from build123d import *

# Parameters (mm, degrees)
SKETCH2_R           = 4.1
SKETCH2_R_2         = 2.6
BOSS_EXTRUDE1_DEPTH = 5


with BuildPart() as part:
    # Sketch2 → Boss-Extrude1 (new body)
    # profile 1 of 2: a face of its own
    with BuildSketch(Plane.XY):
        with BuildLine():
            ThreePointArc((-8.388352144, 2.232508627), (-7.643352144, 2.753972912), (-8.388352144, 3.275437196))
            Line((-8.388352144, 3.275437196), (-8.388352144, 4.232508627))
            ThreePointArc((-8.388352144, 4.232508627), (-7.805907881, 4.361528648), (-7.67688786, 4.943972912))
            Line((-7.67688786, 4.943972912), (-6.719816429, 4.943972912))
            ThreePointArc((-6.719816429, 4.943972912), (-6.198352144, 4.198972912), (-5.67688786, 4.943972912))
            Line((-5.67688786, 4.943972912), (-4.719816429, 4.943972912))
            ThreePointArc((-4.719816429, 4.943972912), (-4.198352144, 4.198972912), (-3.67688786, 4.943972912))
            Line((-3.67688786, 4.943972912), (-2.719816429, 4.943972912))
            ThreePointArc((-2.719816429, 4.943972912), (-2.198352144, 4.198972912), (-1.67688786, 4.943972912))
            Line((-1.67688786, 4.943972912), (-0.719816429, 4.943972912))
            ThreePointArc((-0.719816429, 4.943972912), (-0.198352144, 4.198972912), (0.32311214, 4.943972912))
            Line((0.32311214, 4.943972912), (1.280183571, 4.943972912))
            ThreePointArc((1.280183571, 4.943972912), (1.409203592, 4.361528648), (1.991647856, 4.232508627))
            Line((1.991647856, 4.232508627), (1.991647856, 3.275437196))
            ThreePointArc((1.991647856, 3.275437196), (1.246647856, 2.753972912), (1.991647856, 2.232508627))
            Line((1.991647856, 2.232508627), (1.991647856, 1.275437196))
            ThreePointArc((1.991647856, 1.275437196), (1.246647856, 0.753972912), (1.991647856, 0.232508627))
            Line((1.991647856, 0.232508627), (1.991647856, -0.724562804))
            ThreePointArc((1.991647856, -0.724562804), (1.246647856, -1.246027088), (1.991647856, -1.767491373))
            Line((1.991647856, -1.767491373), (1.991647856, -2.724562804))
            ThreePointArc((1.991647856, -2.724562804), (1.246647856, -3.246027088), (1.991647856, -3.767491373))
            Line((1.991647856, -3.767491373), (1.991647856, -4.724562804))
            ThreePointArc((1.991647856, -4.724562804), (1.409203592, -4.853582824), (1.280183571, -5.436027088))
            Line((1.280183571, -5.436027088), (0.32311214, -5.436027088))
            ThreePointArc((0.32311214, -5.436027088), (-0.198352144, -4.691027088), (-0.719816429, -5.436027088))
            Line((-0.719816429, -5.436027088), (-1.67688786, -5.436027088))
            ThreePointArc((-1.67688786, -5.436027088), (-2.198352144, -4.691027088), (-2.719816429, -5.436027088))
            Line((-2.719816429, -5.436027088), (-3.67688786, -5.436027088))
            ThreePointArc((-3.67688786, -5.436027088), (-4.198352144, -4.691027088), (-4.719816429, -5.436027088))
            Line((-4.719816429, -5.436027088), (-5.67688786, -5.436027088))
            ThreePointArc((-5.67688786, -5.436027088), (-6.198352144, -4.691027088), (-6.719816429, -5.436027088))
            Line((-6.719816429, -5.436027088), (-7.67688786, -5.436027088))
            ThreePointArc((-7.67688786, -5.436027088), (-7.805907881, -4.853582824), (-8.388352144, -4.724562804))
            Line((-8.388352144, -4.724562804), (-8.388352144, -3.767491373))
            ThreePointArc((-8.388352144, -3.767491373), (-7.643352144, -3.246027088), (-8.388352144, -2.724562804))
            Line((-8.388352144, -2.724562804), (-8.388352144, -1.767491373))
            ThreePointArc((-8.388352144, -1.767491373), (-7.643352144, -1.246027088), (-8.388352144, -0.724562804))
            Line((-8.388352144, -0.724562804), (-8.388352144, 0.232508627))
            ThreePointArc((-8.388352144, 0.232508627), (-7.643352144, 0.753972912), (-8.388352144, 1.275437196))
            Line((-8.388352144, 1.275437196), (-8.388352144, 2.232508627))
        make_face()
        with Locations((-3.198352144, -0.246027088)):
            Circle(SKETCH2_R, mode=Mode.SUBTRACT)
    # profile 2 of 2: a face of its own
    with BuildSketch(Plane.XY):
        with Locations((-3.198352144, -0.246027088)):
            Circle(SKETCH2_R)
        with Locations((-3.198352144, -0.246027088)):
            Circle(SKETCH2_R_2, mode=Mode.SUBTRACT)
    extrude(amount=BOSS_EXTRUDE1_DEPTH)


solid = part.part
Verification items for the finished model (mm, model axes). Coordinates: 2 decimals unless noted, no trailing zeros. Order: outer loops, then holes, each group sorted by start corner. A loop starts at its lowest first (then second) coordinate and runs counter-clockwise, first axis right, second up. Notation, with made-up numbers: M 83,-32.75 L 140,-32.75 A21 cw 140,-4.75 Z; hole C -4,37.25 d6. An arc over 180 degrees is marked long. One line per item, written item: value. Start each with the question number.
Item 1: Depth check by flat-ended pin: P1, Ø6, axis at x = -6, y = 0, coming from the -Z side; P2, Ø1, axis at x = -0.2, y = -5.25, coming from the -Z side. Enter the tip coordinate at first touch or a pass-through.
Item 2: Thickness scan on probe 1 along X at (y, z) = (-5, 0.6); probe 2 along Y at (x, z) = (-6, 2.35); probe 3 along X at (y, z) = (-2.25, 3.95). Record the ranges inside material, lowest first.
Item 3: Sectioned sample at A-A on y = 0.5. Record the cut outline in (x, z).
Item 4: Mould release check, pull along X, two halves, no side actions. Record for faces 1 (the cylindrical face through (1.247, -1.231, 2.465)), 2 (the flat face through (-5, -5.436, 2)), 3 (the flat face through (1.992, -2, 2)): pulls with the +X half, pulls with the -X half, needs draft (parallel to the pull), parting line crosses it, or undercut.
Item 5: Sectioned sample at C-C on y = 3. Record the cut outline in (x, z), then the cut area to 3 significant figures.
Item 6: Sectioned sample at B-B on x = -6. Record the cut outline in (y, z), then the cut area to 3 significant figures.
Calculated:
1. P1: z = 0
1. P2: through
2. probe 1: -7.7 to -6.7, -5.7 to -4.7, -3.7 to -2.7, -1.7 to -0.7, 0.3 to 1.3
2. probe 2: -4.73 to 4.24
2. probe 3: -8.39 to -4.85, -1.54 to 1.99
3. outline: M -7.7,0 L -5.69,0 L -5.69,5 L -7.7,5 Z; M -0.71,0 L 1.31,0 L 1.31,5 L -0.71,5 Z
4. face 1: undercut
4. face 2: needs draft
4. face 3: pulls with the +X half
5. outline: M -7.7,0 L 1.3,0 L 1.3,5 L -7.7,5 Z
5. area: 45.0 mm^2
6. outline: M -4.73,0 L 4.24,0 L 4.24,5 L -4.73,5 Z
6. area: 44.8 mm^2
